Model file for the job. Use its own axes, mm. Coordinates: 2 decimals unless noted, no trailing zeros. Order: outer loops, then holes, each group sorted by start corner. A loop starts at its lowest first (then second) coordinate and runs counter-clockwise, first axis right, second up.
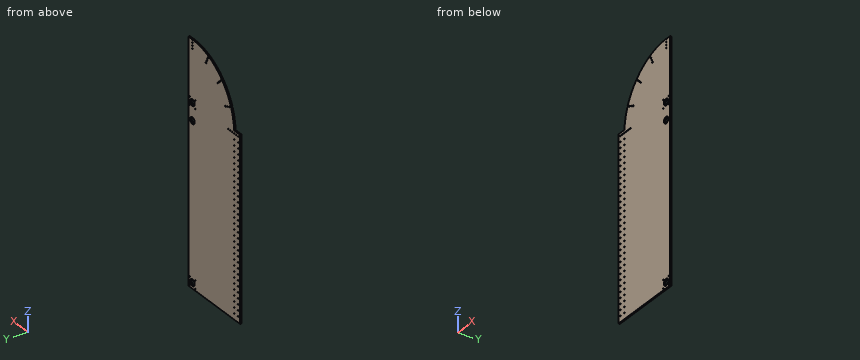
from build123d import *

# Parameters (mm, degrees)
F0_R     = 14.2875
F1_DEPTH = 6.35
F2_R     = 2.5527
F3_DEPTH = 25.4
F4_R     = 2.159
F5_DEPTH = 25.4
F7_D     = 5.1054
F9_DEPTH = 25.4


# Not quite as in the source:
# - a feature names something its author has since deleted; it is built from what else it names


with BuildPart() as f1:
    # F0 (on Front) → F1 (new body)
    with BuildSketch(Plane.XZ):
        Polygon((25.4, -787.4), (25.4, 0), (25.4, 304.8), (-304.8, 304.8), (-304.8, 0), (-304.8, -787.4), align=None)
        with Locations((0, -762)):
            Circle(F0_R, mode=Mode.SUBTRACT)
        with Locations((0, -76.2)):
            Circle(F0_R, mode=Mode.SUBTRACT)
        Circle(F0_R, mode=Mode.SUBTRACT)
    extrude(amount=F1_DEPTH)

    # F2 (on face) → F3 (cut)
    with BuildSketch(Plane.XZ.offset(6.35)):
        with Locations((-292.1, -25.4)):
            Circle(F2_R)
        with Locations((-292.1, -50.8)):
            Circle(F2_R)
        with Locations((-266.7, -50.8)):
            Circle(F2_R)
        with Locations((-266.7, -25.4)):
            Circle(F2_R)
        with Locations((-266.7, 0)):
            Circle(F2_R)
        with Locations((-292.1, 0)):
            Circle(F2_R)
        with Locations((-292.1, -76.2)):
            Circle(F2_R)
        with Locations((-266.7, -76.2)):
            Circle(F2_R)
        with Locations((-292.1, -101.6)):
            Circle(F2_R)
        with Locations((-266.7, -101.6)):
            Circle(F2_R)
        with Locations((-266.7, -127)):
            Circle(F2_R)
        with Locations((-292.1, -127)):
            Circle(F2_R)
        with Locations((-292.1, -152.4)):
            Circle(F2_R)
        with Locations((-266.7, -152.4)):
            Circle(F2_R)
        with Locations((-292.1, -177.8)):
            Circle(F2_R)
        with Locations((-266.7, -177.8)):
            Circle(F2_R)
        with Locations((-266.7, -203.2)):
            Circle(F2_R)
        with Locations((-292.1, -203.2)):
            Circle(F2_R)
        with Locations((-292.1, -228.6)):
            Circle(F2_R)
        with Locations((-266.7, -228.6)):
            Circle(F2_R)
        with Locations((-292.1, -254)):
            Circle(F2_R)
        with Locations((-266.7, -254)):
            Circle(F2_R)
        with Locations((-266.7, -279.4)):
            Circle(F2_R)
        with Locations((-292.1, -279.4)):
            Circle(F2_R)
        with Locations((-292.1, -304.8)):
            Circle(F2_R)
        with Locations((-266.7, -304.8)):
            Circle(F2_R)
        with Locations((-266.7, -330.2)):
            Circle(F2_R)
        with Locations((-292.1, -330.2)):
            Circle(F2_R)
        with Locations((-292.1, -355.6)):
            Circle(F2_R)
        with Locations((-266.7, -355.6)):
            Circle(F2_R)
        with Locations((-266.7, -381)):
            Circle(F2_R)
        with Locations((-292.1, -381)):
            Circle(F2_R)
        with Locations((-266.7, -406.4)):
            Circle(F2_R)
        with Locations((-292.1, -406.4)):
            Circle(F2_R)
        with Locations((-292.1, -431.8)):
            Circle(F2_R)
        with Locations((-266.7, -431.8)):
            Circle(F2_R)
        with Locations((-266.7, -457.2)):
            Circle(F2_R)
        with Locations((-292.1, -457.2)):
            Circle(F2_R)
        with Locations((-266.7, -482.6)):
            Circle(F2_R)
        with Locations((-292.1, -482.6)):
            Circle(F2_R)
        with Locations((-292.1, -508)):
            Circle(F2_R)
        with Locations((-266.7, -508)):
            Circle(F2_R)
        with Locations((-266.7, -533.4)):
            Circle(F2_R)
        with Locations((-292.1, -533.4)):
            Circle(F2_R)
        with Locations((-266.7, -558.8)):
            Circle(F2_R)
        with Locations((-292.1, -558.8)):
            Circle(F2_R)
        with Locations((-292.1, -584.2)):
            Circle(F2_R)
        with Locations((-266.7, -584.2)):
            Circle(F2_R)
        with Locations((-266.7, -609.6)):
            Circle(F2_R)
        with Locations((-292.1, -609.6)):
            Circle(F2_R)
        with Locations((-266.7, -635)):
            Circle(F2_R)
        with Locations((-292.1, -635)):
            Circle(F2_R)
        with Locations((-292.1, -660.4)):
            Circle(F2_R)
        with Locations((-266.7, -660.4)):
            Circle(F2_R)
        with Locations((-266.7, -685.8)):
            Circle(F2_R)
        with Locations((-292.1, -685.8)):
            Circle(F2_R)
        with Locations((-266.7, -711.2)):
            Circle(F2_R)
        with Locations((-292.1, -711.2)):
            Circle(F2_R)
        with Locations((-292.1, -736.6)):
            Circle(F2_R)
        with Locations((-266.7, -736.6)):
            Circle(F2_R)
        with Locations((-266.7, -762)):
            Circle(F2_R)
        with Locations((-292.1, -762)):
            Circle(F2_R)
    extrude(amount=-F3_DEPTH, mode=Mode.SUBTRACT)

    # F4 (on face) → F5 (cut)
    with BuildSketch(Plane.XZ.offset(6.35)):
        with Locations((-17.5, -744.5)):
            Circle(F4_R)
        with Locations((17.5, -744.5)):
            Circle(F4_R)
        with Locations((17.5, -779.5)):
            Circle(F4_R)
        with Locations((-17.5, -779.5)):
            Circle(F4_R)
        with Locations((17.5, -17.5)):
            Circle(F4_R)
        with Locations((17.5, 17.5)):
            Circle(F4_R)
        with Locations((-17.5, 17.5)):
            Circle(F4_R)
        with Locations((-17.5, -17.5)):
            Circle(F4_R)
    extrude(amount=-F5_DEPTH, mode=Mode.SUBTRACT)

    # F7 (through all)
    with Locations(Plane.XZ.offset(6.35)):
        with Locations((-87.4814326387, 211.1988611321), (-92.3415122297, 222.932131195), (-97.2015918207, 234.6654012579), (-102.0616714118, 246.3986713208), (-106.9217510028, 258.1319413837), (0, 266.7), (0, 254), (0, 241.3), (0, 228.6), (0, 279.4), (-266.7, 0), (-254, 0), (-279.4, 0), (-258.1319413837, 106.9217510028), (-246.3986713208, 102.0616714118), (-234.6654012579, 97.2015918207), (-241.3, 0), (-228.6, 0), (-222.932131195, 92.3415122297), (-161.6446101792, 161.6446101792), (-170.6248663003, 170.6248663003), (-188.5853785425, 188.5853785425), (-179.6051224214, 179.6051224214), (-211.1988611321, 87.4814326387), (-197.5656346635, 197.5656346635)):
            Hole(F7_D / 2)

    # F8 (on face) → F9 (cut)
    with BuildSketch(Plane.XZ.offset(6.35)):
        with BuildLine():
            Line((-304.8, 304.8), (-304.8, 12.7))
            Line((-304.8, 12.7), (-266.7, 12.7))
            ThreePointArc((-266.7, 12.7), (-184.2542427414, 193.2370410449), (0, 267.0022097287))
            Line((0, 267.0022097287), (25.4, 267.0022097287))
            Line((25.4, 267.0022097287), (25.4, 304.8))
            Line((25.4, 304.8), (-304.8, 304.8))
        make_face()
    extrude(amount=-F9_DEPTH, mode=Mode.SUBTRACT)


solid = f1.part
Q1. Probe line 1 (X direction, y = -1.25, z = -762); line 2 (Z direction, x = -102, y = -4.5); line 3 (X direction, y = -3.5, z = 143). List the from-to ranges inside material, lowest first.
Established:
line 1: x = -304.8 to -294.65, -289.55 to -269.25, -264.15 to -14.29, 14.29 to 25.4
line 2: z = -787.4 to 243.85
line 3: x = -225.48 to 25.4
Q2. Drop flat-ended pins along their axis: P1, Ø4, axis at x = -234.67, z = 97.2, coming from the +Y side; P2, Ø1, axis at x = -56, y = -2, coming from the +Z side. Give the stop position or say it passes through.
Established:
P1: passes through
P2: stops at z = 261.17
Q3. Cut at B-B, the plane x = -135.5. List the corners of the cut face in (y, z).
Established:
outline: (-6.35, -787.4) - (0, -787.4) - (0, 230.07) - (-6.35, 230.07) - close
Q4. Cut at A-A, the plane y = -5.25. Count the separate pieces of the cut face and the enclosed holes in it, plus the area to 3 significant figures.
Established:
separate pieces: 1
enclosed holes: 89
area: 320,000 mm2
